Here's how the part is built. I have some questions about the finished solid (model axes, mm). Face numbers are marked on the shaded views. A direction names the side the tool comes from. Round coordinates to 2 decimals unless told otherwise and drop trailing zeros. Order: outer loops, then holes, each group sorted by start corner. A loop starts at its lowest first (then second) coordinate and runs counter-clockwise, first axis right, second up. Notation, with made-up numbers: (24.5, 61) -> (51.5, 61) arc R27 cw to (51.5, 94) -> close; hole circle Ø10 at (-8.75, 41). An arc over 180 degrees is marked (long way). Use a Markdown table: item, result. Add a question column.
(1) If I drill on probe 1 along X at (y, z) = (77.5, -63); probe 2 along Z at (x, y) = (-9, 78); probe 3 along Z at (x, y) = (41, 224.5), over which ranges is the centre line in solid material (lowest first)?
(2) I want a section at A-A, the plane z = -82.5. Please give me the cut outline in (x, y), then the cut area to 3 significant figures.
(3) On a 3-axis mill with a long thin cutter (end or side, diameter ignored), from which of +Z, -Z, +X, -X, +Y, -Y can I reach the whole of each face in a straight line? I mean the marked faces 1 and 2. Say none if no direction works.
(4) I want a section at B-B, the plane y = 159. Please give me the cut outline in (x, z).
(5) Thinking about a two-plate mould opening in X: for the marked faces 3, 4 and 5, which applies, pulls with the +X half, pulls with the -X half, needs draft (parallel to the pull), parting line crosses it, or undercut?
from build123d import *

# Parameters (mm, degrees)
F0_W     = 500.126
F0_H     = 228.6
F1_DEPTH = 350.012
F2_R     = 5.08
F4_DEPTH = 350.013
F5_R     = 5.08


with BuildPart() as f1:
    # F0 (on Front) → F1 (new body)
    with BuildSketch(Plane.XZ):
        Rectangle(F0_W, F0_H)
    extrude(amount=-F1_DEPTH)

    # F2
    f2_edges = [f1.edges().sort_by_distance(p)[0] for p in [
        (0, 0, -114.3),
        (250.063, 0, 0),
        (0, 0, 114.3),
        (-250.063, 0, 0),
        (-250.063, 175.006, 114.3),
        (-250.063, 175.006, -114.3),
        (-250.063, 350.012, 0),
        (250.063, 175.006, 114.3),
        (0, 350.012, 114.3),
        (250.063, 175.006, -114.3),
        (0, 350.012, -114.3),
        (250.063, 350.012, 0),
    ]]
    fillet(f2_edges, radius=F2_R)

    # F3 (on face) → F4 (cut, through all)
    with BuildSketch(Plane(origin=(0, 350.012, 0), x_dir=(-1, 0, 0), z_dir=(0, 1, 0))):
        Polygon((38.1, -94.107), (38.1, -45.6269201875), (0, -45.6269201875), (-38.1, -45.6269201875), (-38.1, -121.8269201875), (0, -121.8269201875), (38.1, -121.8269201875), align=None)
    extrude(amount=-F4_DEPTH, mode=Mode.SUBTRACT)

    # F5
    f5_edges = [f1.edges().sort_by_distance(p)[0] for p in [
        (0, 0, -45.62692),
        (-38.1, 0, -77.42346),
        (38.1, 0, -77.42346),
        (-38.1, 350.012, -77.42346),
        (0, 350.012, -45.62692),
        (38.1, 350.012, -77.42346),
        (-38.1, 175.006, -114.3),
        (-38.1, 1.487898, -112.812102),
        (-38.1, 348.524102, -112.812102),
        (38.1, 1.487898, -112.812102),
        (38.1, 348.524102, -112.812102),
        (38.1, 175.006, -114.3),
    ]]
    fillet(f5_edges, radius=F5_R)


solid = f1.part
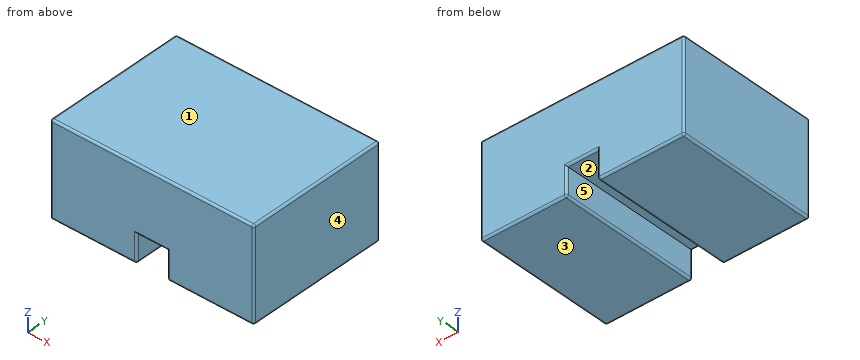
Taken from the geometry:
| question | item | result |
|---|---|---|
| 1 | probe 1 | x = -250.06 to -38.1, 38.1 to 250.06 |
| 1 | probe 2 | z = -45.63 to 114.3 |
| 1 | probe 3 | z = -113.81 to 114.3 |
| 2 | outline | (-250.06, 5.08) arc R5.08 ccw to (-244.98, 0) -> (-43.18, 0) arc R5.08 ccw to (-38.1, 5.08) -> (-38.1, 344.93) arc R5.08 ccw to (-43.18, 350.01) -> (-244.98, 350.01) arc R5.08 ccw to (-250.06, 344.93) -> close; (38.1, 5.08) arc R5.08 ccw to (43.18, 0) -> (244.98, 0) arc R5.08 ccw to (250.06, 5.08) -> (250.06, 344.93) arc R5.08 ccw to (244.98, 350.01) -> (43.18, 350.01) arc R5.08 ccw to (38.1, 344.93) -> close |
| 2 | area | 148,000 mm2 |
| 3 | face 1 | +Z, +X, -X, +Y, -Y |
| 3 | face 2 | -Z, +Y, -Y |
| 4 | outline | (-250.06, -109.22) arc R5.08 ccw to (-244.98, -114.3) -> (-43.18, -114.3) arc R5.08 ccw to (-38.1, -109.22) -> (-38.1, -45.63) -> (38.1, -45.63) -> (38.1, -109.22) arc R5.08 ccw to (43.18, -114.3) -> (244.98, -114.3) arc R5.08 ccw to (250.06, -109.22) -> (250.06, 109.22) arc R5.08 ccw to (244.98, 114.3) -> (-244.98, 114.3) arc R5.08 ccw to (-250.06, 109.22) -> close |
| 5 | face 3 | needs draft |
| 5 | face 4 | pulls with the +X half |
| 5 | face 5 | undercut |
